Build history of the part. All positions in model axes, mm. Face numbers are marked on the shaded views. A direction names the side the tool comes from. Round coordinates to 2 decimals unless told otherwise and drop trailing zeros. Loops run counter-clockwise (first coordinate to the right, second up) from the corner with the lowest first, then second, coordinate; pieces in that order, holes last.
from build123d import *

# Parameters (mm, degrees)
SKETCH1_R           = 9
BOSS_EXTRUDE1_DEPTH = 50
SKETCH2_R           = 5
BOSS_EXTRUDE2_DEPTH = 2
SKETCH4_W           = 12
SKETCH4_H           = 12
SKETCH4_R           = 5
BOSS_EXTRUDE3_DEPTH = 1


with BuildPart() as part:
    # Sketch1 → Boss-Extrude1 (new body)
    with BuildSketch(Plane.XY):
        Circle(SKETCH1_R)
    extrude(amount=-BOSS_EXTRUDE1_DEPTH)



with BuildPart() as body_2:
    # Sketch2 → Boss-Extrude2 (new body)
    with BuildSketch(Plane.XY):
        with BuildLine():
            Line((0, 0), (0, 6))
            Line((0, 6), (70, 6))
            ThreePointArc((70, 6), (76, 0), (70, -6))
            Line((70, -6), (0, -6))
            Line((0, -6), (0, 0))
        make_face()
        with Locations((70, 0)):
            Circle(SKETCH2_R, mode=Mode.SUBTRACT)
    extrude(amount=BOSS_EXTRUDE2_DEPTH)


with BuildPart() as part_1:
    add(part.part)

    add(body_2.part)  # Boss-Extrude3 merges body 2
    # Sketch4 → Boss-Extrude3 (add, symmetric)
    with BuildSketch(Plane(origin=(0, 0, 0), x_dir=(1, 0, 0), z_dir=(0, 1, 0))):
        with Locations((0, -6)):
            Rectangle(SKETCH4_W, SKETCH4_H)
        with BuildLine():
            Line((-6, -12), (-6, 0))
            Line((-6, 0), (-24, 0))
            ThreePointArc((-24, 0), (-30, -6), (-24, -12))
            Line((-24, -12), (-6, -12))
        make_face()
        with Locations((-24, -6)):
            Circle(SKETCH4_R, mode=Mode.SUBTRACT)
        with BuildLine():
            Line((6, -12), (-6, -12))
            Line((-6, -12), (-6, -30))
            ThreePointArc((-6, -30), (0, -36), (6, -30))
            Line((6, -30), (6, -12))
        make_face()
        with Locations((0, -30)):
            Circle(SKETCH4_R, mode=Mode.SUBTRACT)
    extrude(amount=BOSS_EXTRUDE3_DEPTH, both=True)


solid = part_1.part
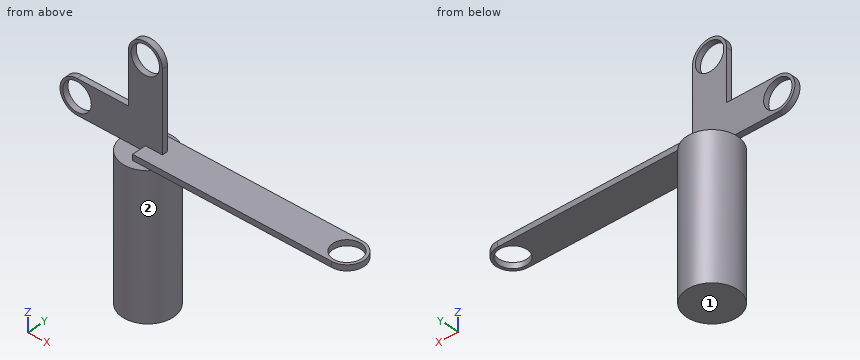
(1) Slice it at D-D on z = 15. List the corners of the cut face in (x, y), plus the area to 3 significant figures.
Responses:
outline: (-6, -1) - (6, -1) - (6, 1) - (-6, 1) - close
area: 24.0 mm2
(2) Probe line 1 (Z direction, x = 0, y = 0.4); line 2 (X direction, y = 0.35, z = 30); line 3 (X direction, y = -0.05, z = 6). List the from-to ranges inside material, lowest first.
Responses:
line 1: z = -50 to 25, 35 to 36
line 2: x = -6 to -5, 5 to 6
line 3: x = -30 to -29, -19 to 6
(3) Slice it at B-B on x = 67.5. List the corners of the cut face in (y, z), plus the area to 3 significant figures.
Responses:
outline: (-6, 0) - (-4.33, 0) - (-4.33, 2) - (-6, 2) - close; (4.33, 0) - (6, 0) - (6, 2) - (4.33, 2) - close
area: 6.68 mm2
(4) Slice it at C-C on y = -3. List the corners of the cut face in (x, z), plus the area to 3 significant figures.
Responses:
outline: (-8.49, -50) - (8.49, -50) - (8.49, 0) - (66, 0) - (66, 2) - (0, 2) - (0, 0) - (-8.49, 0) - close; (74, 0) - (75.2, 0) - (75.2, 2) - (74, 2) - close
area: 983 mm2
(5) Pin check, flat tips, straight feed: P1, Ø5, axis at y = -4.5, z = -17, coming from the -X side; P2, Ø1, axis at x = -12, y = 0, coming from the +Z side; P3, Ø0.6, axis at x = 48, z = 1.5, coming from the -Y side. Stop position of each tip, or through.
Responses:
P1: stops at x = -8.77
P2: stops at z = 12
P3: stops at y = -6
(6) Which spindle directions (+Z, -Z, +X, -X, +Y, -Y) get a long thin tool onto all of the face, cutting with end or side? Do the marked faces 1 and 2. Say none if no direction does.
Responses:
face 1: -Z, +X, -X, +Y, -Y
face 2: -Z
(7) Slice it at A-A on z = 6. List the corners of the cut face in (x, y).
Responses:
outline: (-30, -1) - (-29, -1) - (-29, 1) - (-30, 1) - close; (-19, -1) - (6, -1) - (6, 1) - (-19, 1) - close
